Geometry: see drawing. Coordinates: mm, zero at the bounding-box minimum. A direction names the side the tool comes from. Give positions to 0.01 mm unless a question says otherwise; leave off trailing zeros. Loops run counter-clockwise (first coordinate to the right, second up) from the corner with the lowest first, then second, coordinate; pieces in that order, holes last. Notation, with made-up numbers: M 36.5,62.25 L 48.5,62.25 A16 cw 48.5,76.25 Z; hole C -15.75,80.25 d6. An arc over 180 degrees is marked long. Put each result on its own line as item: value.
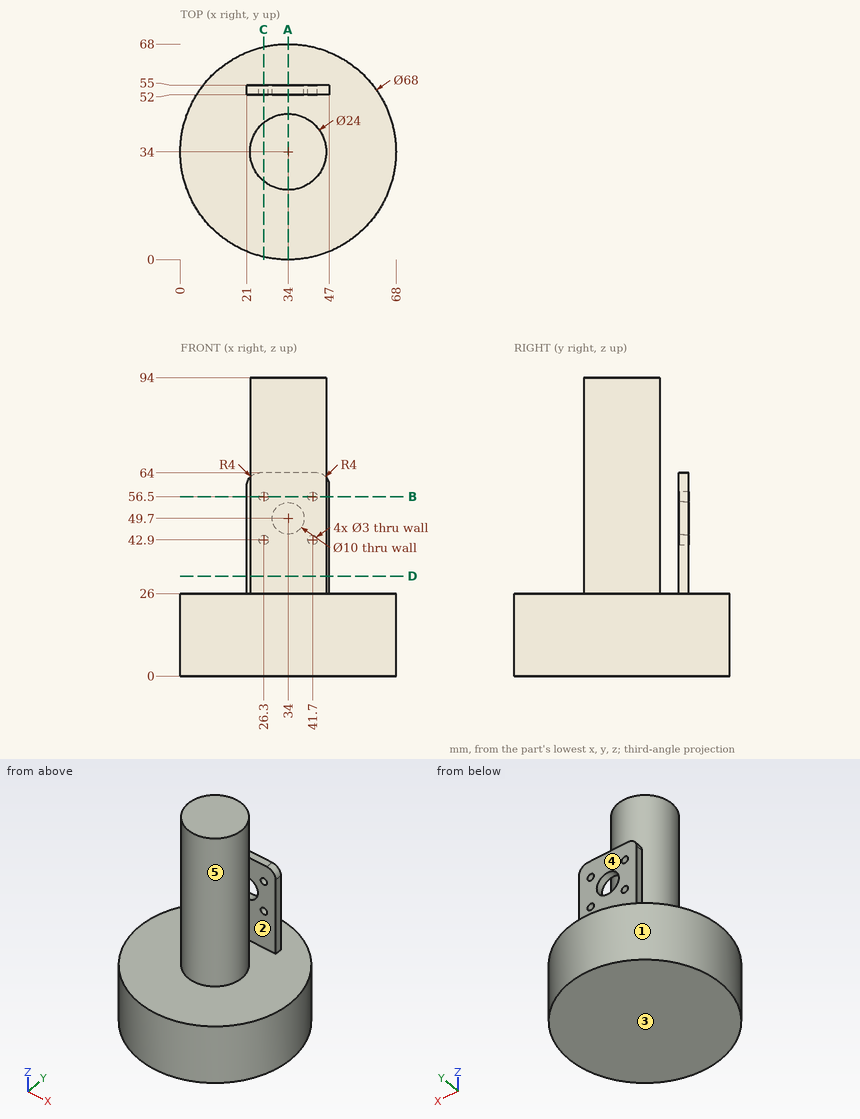
Item 1: Section B-B on z = 56.5. Output: boundary loops of the cut face in (x, y).
Output values:
outline: M 21,52 L 24.8,52 L 24.8,55 L 21,55 Z; C 34,34 d24; M 27.8,52 L 40.2,52 L 40.2,55 L 27.8,55 Z; M 43.2,52 L 47,52 L 47,55 L 43.2,55 Z
Item 2: Pin query (flat end, axial travel): pin 1 Ø2.5 at (x, y) = (35, 53) entering from +Z; pin 2 Ø8 at (x, z) = (37, 46) entering from +Y; pin 3 Ø21 at (x, z) = (31, 52.5) entering from -Y; pin 4 Ø10 at (x, y) = (55, 24) entering from -Z. Return the tip coordinate at first contact, or that it passes through.
Output values:
pin 1: z = 64
pin 2: y = 55
pin 3: y = 22
pin 4: z = 0
Item 3: Line query: probe 1 along X at (y, z) = (52.65, 42.9); probe 2 along Z at (x, y) = (41, 54); probe 3 along Z at (x, y) = (26, 53). Output: solid intervals per line, ascending. Write a range as [from, to].
Output values:
probe 1: [21, 24.8], [27.8, 40.2], [43.2, 47]
probe 2: [0, 41.57], [44.23, 55.17], [57.83, 64]
probe 3: [0, 41.43], [44.37, 55.03], [57.97, 64]
Item 4: Set-up query: the marked faces 1 and 2. Return all of +Z, -Z, +X, -X, +Y, -Y with unobstructed straight access to the full face (end or side cutting, diameter ignored); none if empty.
Output values:
face 1: +Z, -Z
face 2: +Z, +X, -X
Item 5: Mould query, pull axis Y, two halves, no side actions, for the marked faces 3, 4 and 5. Classes: pulls with the +Y half, pulls with the -Y half, needs draft (parallel to the pull), parting line crosses it, or undercut.
Output values:
face 3: needs draft
face 4: pulls with the +Y half
face 5: undercut
Item 6: Section D-D on z = 31.5. Output: boundary loops of the cut face in (x, y), then the cut area to 3 significant figures.
Output values:
outline: M 21,52 L 47,52 L 47,55 L 21,55 Z; C 34,34 d24
area: 530 mm²
Item 7: Section C-C on x = 26.3. Output: boundary loops of the cut face in (y, z).
Output values:
outline: M 0.88,0 L 67.12,0 L 67.12,26 L 55,26 L 55,41.4 L 52,41.4 L 52,26 L 43.2,26 L 43.2,94 L 24.8,94 L 24.8,26 L 0.88,26 Z; M 52,44.4 L 55,44.4 L 55,55 L 52,55 Z; M 52,58 L 55,58 L 55,64 L 52,64 Z
Item 8: Section A-A on x = 34. Output: boundary loops of the cut face in (y, z), then the cut area to 3 significant figures.
Output values:
outline: M 0,0 L 68,0 L 68,26 L 55,26 L 55,44.7 L 52,44.7 L 52,26 L 46,26 L 46,94 L 22,94 L 22,26 L 0,26 Z; M 52,54.7 L 55,54.7 L 55,64 L 52,64 Z
area: 3,480 mm²
